Input: dimensioned drawing with shaded views. Units: mm. Origin: part minimum x, y, z. A direction names the side the tool comes from. Round coordinates to 2 decimals unless told otherwise and drop trailing zeros. Loops run counter-clockwise (first coordinate to the right, second up) from the corner with the lowest first, then second, coordinate; pieces in that order, holes last.
1) Section C-C, the plane y = 3.5. Return loops of the section in (x, z).
2) Draft query along X for the marked faces 1, 2, 3 and 4. Return one class per face: pulls with the +X half, pulls with the -X half, needs draft (parallel to the pull), parting line crosses it, or undercut.
3) Access query for the marked faces 5, 6, 7, 8 and 9. Directions: +Z, -Z, +X, -X, +Y, -Y. A direction counts if a zero-diameter tool reaches every point of the face in a straight line with its end or side. Return the directions, or none.
4) First-contact query: pin 1 (2 mm diameter, centred on x = 32, z = 3, fed in from +Y); pin 2 (3 mm diameter, centred on y = 4, z = 6, fed in from -X); pin 3 (2 mm diameter, centred on x = 26.5, z = 10, fed in from +Y). Flat tips, straight axial feed; report the tip coordinate or a pass-through.
5) Ray query, line 1 along X through (y, z) = (8.75, 2); line 2 along Z through (x, y) = (30.5, 2.2); line 3 along Y through (x, z) = (5.5, 8.25). Return the intervals inside material, ascending.
6) Section A-A, the plane x = 30.5. Return loops of the section in (y, z).
7) Section B-B, the plane z = 5.5. Return loops of the section in (x, y), and give its area (3 significant figures).
8) Section D-D, the plane z = 8.5. Return loops of the section in (x, y).
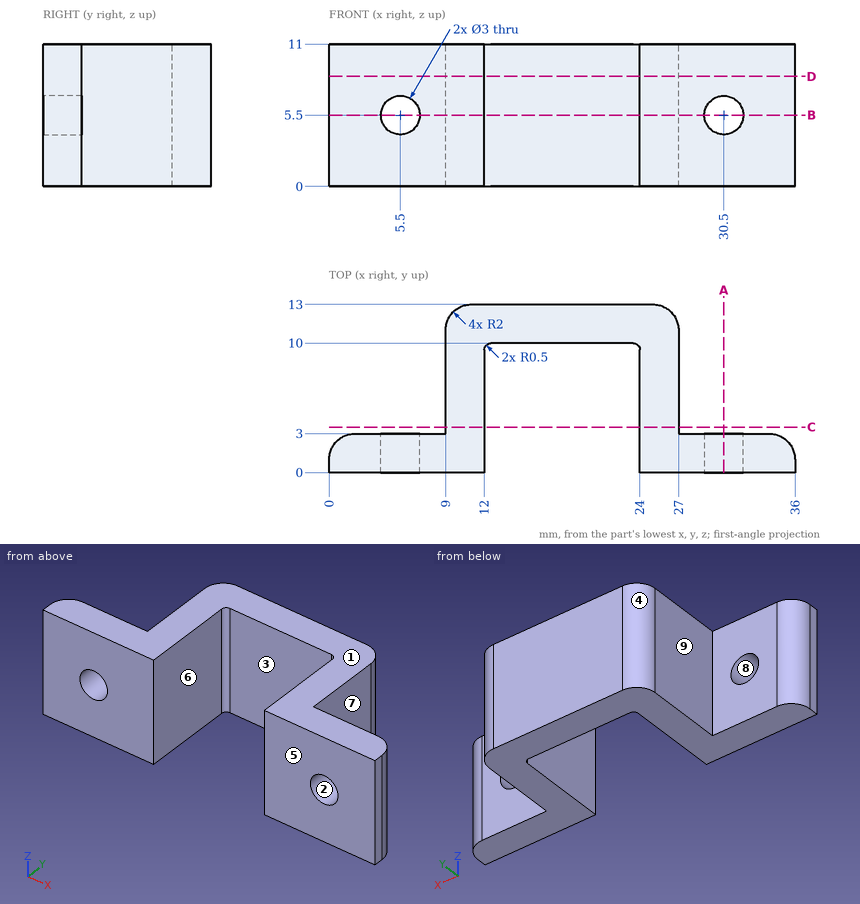
Final values:
1. outline: (9, 0) - (12, 0) - (12, 11) - (9, 11) - close; (24, 0) - (27, 0) - (27, 11) - (24, 11) - close
2. face 1: needs draft
2. face 2: undercut
2. face 3: undercut
2. face 4: pulls with the -X half
3. face 5: +Z, -Z, +X, -X, -Y
3. face 6: +Z, -Z, -Y
3. face 7: +Z, -Z, +X, +Y
3. face 8: +Y, -Y
3. face 9: +Z, -Z, -X, +Y
4. pin 1: stops at y = 3
4. pin 2: stops at x = 0.68
4. pin 3: stops at y = 12.94
5. line 1: x = 9 to 12, 24 to 27
5. line 2: z = 0 to 4, 7 to 11
5. line 3: y = 0 to 3
6. outline: (0, 0) - (3, 0) - (3, 4) - (0, 4) - close; (0, 7) - (3, 7) - (3, 11) - (0, 11) - close
7. outline: (0, 0) - (4, 0) - (4, 3) - (2, 3) arc R2 ccw to (0, 1) - close; (7, 0) - (12, 0) - (12, 9.5) arc R0.5 cw to (12.5, 10) - (23.5, 10) arc R0.5 cw to (24, 9.5) - (24, 0) - (29, 0) - (29, 3) - (27, 3) - (27, 11) arc R2 ccw to (25, 13) - (11, 13) arc R2 ccw to (9, 11) - (9, 3) - (7, 3) - close; (32, 0) - (36, 0) - (36, 1) arc R2 ccw to (34, 3) - (32, 3) - close
7. area: 147 mm2
8. outline: (0, 0) - (12, 0) - (12, 9.5) arc R0.5 cw to (12.5, 10) - (23.5, 10) arc R0.5 cw to (24, 9.5) - (24, 0) - (36, 0) - (36, 1) arc R2 ccw to (34, 3) - (27, 3) - (27, 11) arc R2 ccw to (25, 13) - (11, 13) arc R2 ccw to (9, 11) - (9, 3) - (2, 3) arc R2 ccw to (0, 1) - close
